For this review, take the finished solid that the model builds, in its own axes (mm). A direction names the side the tool comes from. Give positions to 0.01 mm unless a question says otherwise; leave off trailing zeros. Loops run counter-clockwise (first coordinate to the right, second up) from the corner with the lowest first, then second, coordinate; pieces in that order, holes last. Notation, with made-up numbers: M -21.5,72 L 26.5,72 A23 ccw 26.5,96 Z; hole C 16,79.25 d9. An arc over 180 degrees is marked long. Use CSV: the item, a comma, the result in double quotes. Start each with the question number.
1. Take a section at D-D, the plane y = -34. Write out the cut boundary in (x, z), and give its area (3 significant figures).
2. To check wall thickness, follow line 1 (Y direction, x = -42.5, z = 38); line 2 (Z direction, x = 4, y = -37); line 3 (Y direction, x = 38, z = 45.5). State the ranges of each line that lie inside material, in increasing order. Write a range as [from, to].
3. Take a section at B-B, the plane y = 30.5. Write out the cut boundary in (x, z) (3 decimals).
4. Take a section at A-A, the plane z = 28. Write out the cut boundary in (x, y).
5. Insertion check: P1, Ø1.5, axis at x = 23, y = 32.5, coming from the +Z side; P2, Ø7.5, axis at y = -41.5, z = 32, coming from the -X side; P3, Ø20.5, axis at x = -2.5, z = 35.5, coming from the -Y side. Each pin has a flat end and moves straight along its axis. Give the tip position at first contact, or say it passes through.
6. Tool access review of faces 1 (the face through (-1, 50.8, 1)), 2 (the face through (26.489, -38, 37)), 3 (the face through (15.31, 38.28, 36.83)): name each direction out of +Z, -Z, +X, -X, +Y, -Y from which nothing blocks a thin tool from reaching the whole face with its end or side.
7. Take a section at C-C, the plane x = 0. Write out the cut boundary in (y, z), and give its area (3 significant figures).
from build123d import *

# Parameters (mm, degrees)
F0_W     = 99.4218587875
F0_H     = 99.4218587875
F1_DEPTH = 50.8
F2_W     = 76.2
F2_H     = 25.4
F3_DEPTH = 25.4
F5_DEPTH = 25.4


with BuildPart() as f1:
    # F0 (on Front) → F1 (new body, symmetric)
    with BuildSketch(Plane.XZ):
        Rectangle(F0_W, F0_H)
    extrude(amount=F1_DEPTH, both=True)

    # F2 (on face) → F3 (cut)
    with BuildSketch(Plane.XZ.offset(50.8)):
        with Locations((-11.6109293938, 37.0109293938)):
            Rectangle(F2_W, F2_H)
    extrude(amount=-F3_DEPTH, mode=Mode.SUBTRACT)

    # F4 (on face) → F5 (cut)
    with BuildSketch(Plane(origin=(0, 50.8, 0), x_dir=(-1, 0, 0), z_dir=(0, 1, 0))):
        Polygon((-49.7109293938, 24.3109293938), (20.0749970604, 49.7109293938), (-49.7109293938, 49.7109293938), align=None)
    extrude(amount=-F5_DEPTH, mode=Mode.SUBTRACT)


solid = f1.part
Result set:
1,outline,"M -49.71,-49.71 L 49.71,-49.71 L 49.71,49.71 L 26.49,49.71 L 26.49,24.31 L -49.71,24.31 Z"
1,area,"7,950 mm2"
2,line 1,"[-25.4, 50.8]"
2,line 2,"[-49.71, 24.31]"
2,line 3,"[-50.8, 25.4]"
3,outline,"M -49.711,-49.711 L 49.711,-49.711 L 49.711,24.311 L -20.075,49.711 L -49.711,49.711 Z"
4,outline,"M -49.71,-25.4 L 26.49,-25.4 L 26.49,-50.8 L 49.71,-50.8 L 49.71,25.4 L 39.58,25.4 L 39.58,50.8 L -49.71,50.8 Z"
5,P1,"z = 34.31"
5,P2,"x = 26.49"
5,P3,"y = -25.4"
6,face 1,"+Z, -Z, +X, -X, +Y"
6,face 2,"+Z, -X, -Y"
6,face 3,"+Z, +X, +Y"
7,outline,"M -50.8,-49.71 L 50.8,-49.71 L 50.8,42.4 L 25.4,42.4 L 25.4,49.71 L -25.4,49.71 L -25.4,24.31 L -50.8,24.31 Z"
7,area,"9,270 mm2"
